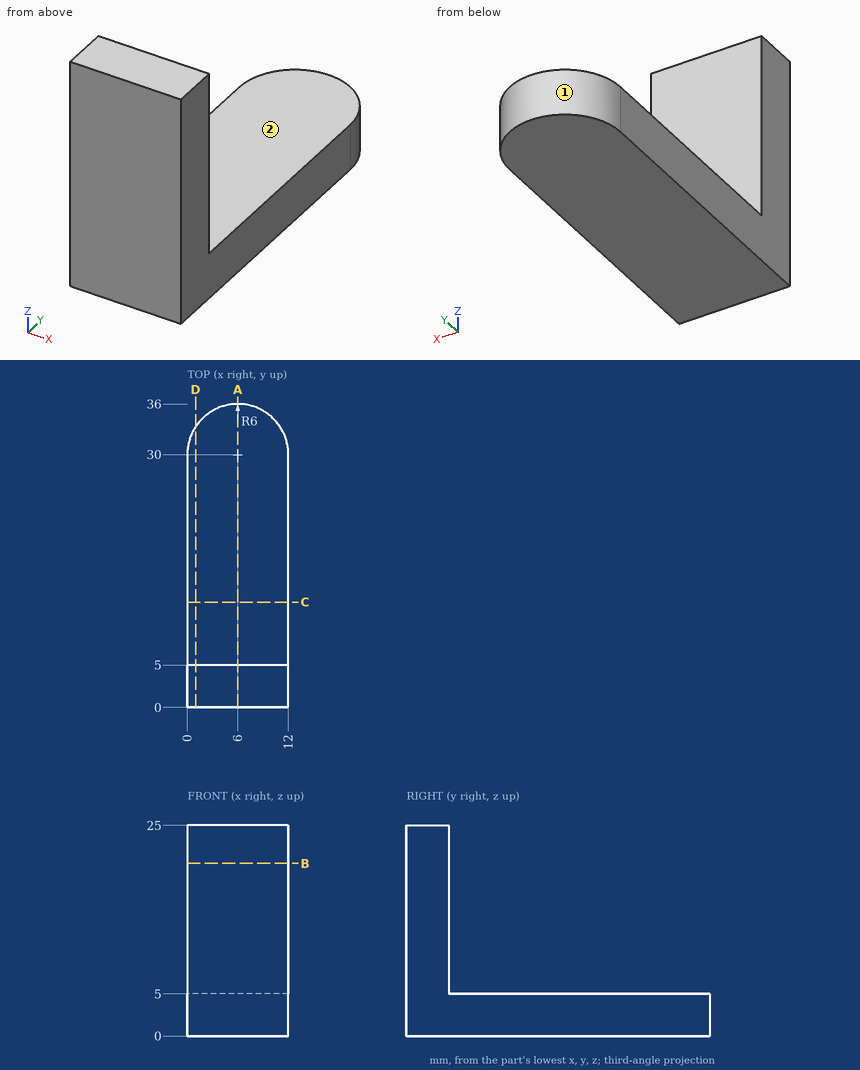
Job drawing, mm, ordinate dimensions from the low corner. One solid piece. A direction names the side the tool comes from. Coordinates: 2 decimals unless noted, no trailing zeros. Loops run counter-clockwise (first coordinate to the right, second up) from the corner with the lowest first, then second, coordinate; pieces in that order, holes last. Notation, with made-up numbers: (6.5, 78.5) - (11.5, 78.5) arc R22 cw to (11.5, 89.5) - close; hole circle Ø11 at (-34, 83). An arc over 180 degrees is marked (long way). Answer as a JSON object with one key per item and string values. Group by question number.
(1) Cut at D-D (x = 1). Give the cut face in (y, z), then the cut area to 3 significant figures.
(2) Tool access for the marked faces 1 and 2: list every direction of +Z, -Z, +X, -X, +Y, -Y with a clear straight run to the whole face (end or side of a thin tool).
(3) Cut at B-B (z = 20.5). Give the cut face in (x, y), then the cut area to 3 significant figures.
(4) Cut at A-A (x = 6). Give the cut face in (y, z), then the cut area to 3 significant figures.
(5) Probe line 1 along Y through (x, z) = (11, 14.75); line 2 along Y through (x, z) = (11, 2.75). List the from-to ranges inside material, lowest first.
(6) Flat gauge pins, fed straight in: pin 1 (4 mm diameter, centred on x = 2.5, z = 13.5, fed in from +Y); pin 2 (6 mm diameter, centred on x = 4.5, y = 25, fed in from +Z). Where does each tip first touch, or does it go through?
Geometry says:
{
 "1": {"outline": "(0, 0) - (33.32, 0) - (33.32, 5) - (5, 5) - (5, 25) - (0, 25) - close", "area": "267 mm^2"},
 "2": {"face 1": "+Z, -Z, +Y", "face 2": "+Z, +X, -X, +Y"},
 "3": {"outline": "(0, 0) - (12, 0) - (12, 5) - (0, 5) - close", "area": "60.0 mm^2"},
 "4": {"outline": "(0, 0) - (36, 0) - (36, 5) - (5, 5) - (5, 25) - (0, 25) - close", "area": "280 mm^2"},
 "5": {"line 1": "y = 0 to 5", "line 2": "y = 0 to 33.32"},
 "6": {"pin 1": "stops at y = 5", "pin 2": "stops at z = 5"}
}
